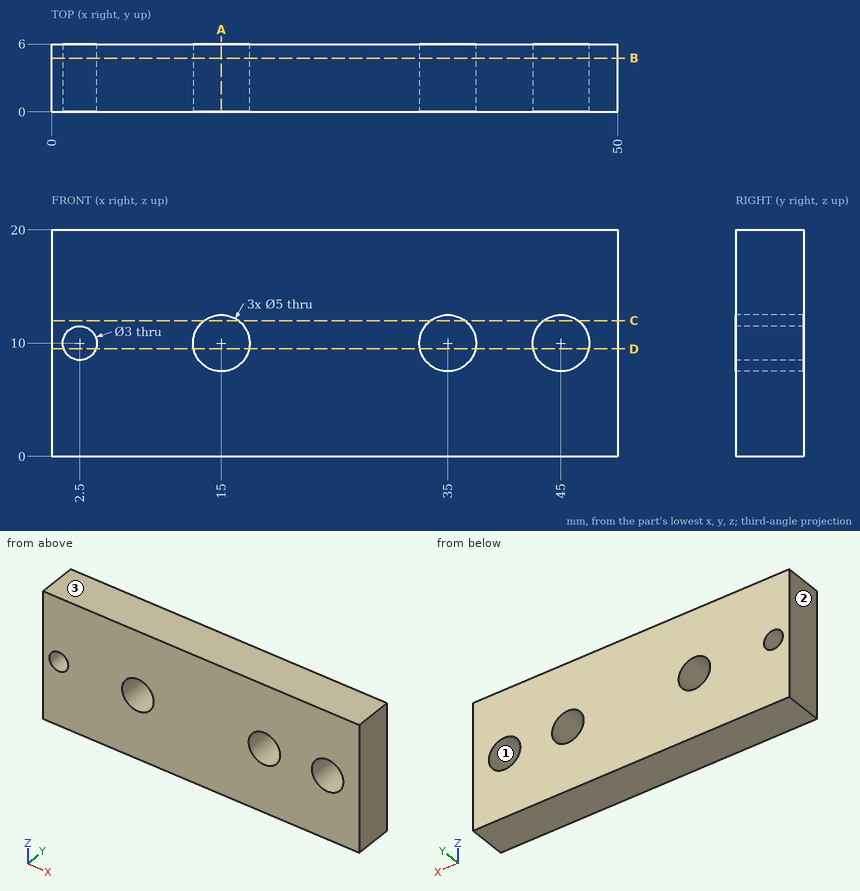
For this review, use the dimensioned drawing (mm, ordinates from the lowest corner) and the shaded views. Give positions to 0.01 mm unless a question says otherwise; leave off trailing zeros. Order: outer loops, then holes, each group sorted by start corner. A loop starts at its lowest first (then second) coordinate and runs counter-clockwise, first axis right, second up. Notation, with made-up numbers: (10, 29.25) - (59, 29.25) arc R22 cw to (59, 35.25) - close; hole circle Ø7 at (25.25, 44.5). An arc over 180 degrees is marked (long way). Write item = value, one per line. Start each with the question number.
Q1. Mouldability with a two-part tool opening along Z and no side actions: class the marked faces 1, 2 and 3 as released by +Z, released by -Z, zero draft, split by the parting line, or undercut.
Q2. We need section D-D on z = 9.5. State the section outline as (x, y) points.
Q3. We need section A-A on x = 15. State the section outline as (y, z) points, plus the area to 3 significant figures.
Q4. We need section C-C on z = 12. State the section outline as (x, y) points, plus the area to 3 significant figures.
Q5. To check wall thickness, follow L1, parallel to X at y = 1.25, z = 10; L2, parallel to Z at x = 2.5, y = 2.85; L3, parallel to X at y = 5.1, z = 7.75. State the ranges of each line that lie inside material, in increasing order. Write a range as from..to.
Q6. Clearance check with a flat-ended pin moving along its axis: pin 1 Ø4 at (x, z) = (35, 10) entering from +Y. State where the tip first meets the part, or that it passes through.
Q7. We need section B-B on y = 4.75. State the section outline as (x, z) points.
Working result:
q1.face_1 = undercut
q1.face_2 = zero draft
q1.face_3 = released by +Z
q2.outline = (0, 0) - (1.09, 0) - (1.09, 6) - (0, 6) - close; (3.91, 0) - (12.55, 0) - (12.55, 6) - (3.91, 6) - close; (17.45, 0) - (32.55, 0) - (32.55, 6) - (17.45, 6) - close; (37.45, 0) - (42.55, 0) - (42.55, 6) - (37.45, 6) - close; (47.45, 0) - (50, 0) - (50, 6) - (47.45, 6) - close
q3.outline = (0, 0) - (6, 0) - (6, 7.5) - (0, 7.5) - close; (0, 12.5) - (6, 12.5) - (6, 20) - (0, 20) - close
q3.area = 90.0 mm²
q4.outline = (0, 0) - (13.5, 0) - (13.5, 6) - (0, 6) - close; (16.5, 0) - (33.5, 0) - (33.5, 6) - (16.5, 6) - close; (36.5, 0) - (43.5, 0) - (43.5, 6) - (36.5, 6) - close; (46.5, 0) - (50, 0) - (50, 6) - (46.5, 6) - close
q4.area = 246 mm²
q5.L1 = 0..1, 4..12.5, 17.5..32.5, 37.5..42.5, 47.5..50
q5.L2 = 0..8.5, 11.5..20
q5.L3 = 0..13.91, 16.09..33.91, 36.09..43.91, 46.09..50
q6.pin_1 = through
q7.outline = (0, 0) - (50, 0) - (50, 20) - (0, 20) - close; hole circle Ø3 at (2.5, 10); hole circle Ø5 at (15, 10); hole circle Ø5 at (35, 10); hole circle Ø5 at (45, 10)
